The model under review builds one solid part; all positions refer to its coordinate system, in mm. Coordinates: 2 decimals unless noted, no trailing zeros. Write each loop counter-clockwise with the first axis right and the second up, starting at its lowest first coordinate (ties: lowest second). Pieces come first, ordered by that corner, then holes. Notation, with made-up numbers: M 39,-13 L 63,-13 A9 cw 63,-7 Z; hole C 83,25.5 d1. An arc over 180 degrees is marked long. Answer as CSV lines item,"result". Start each with the question number.
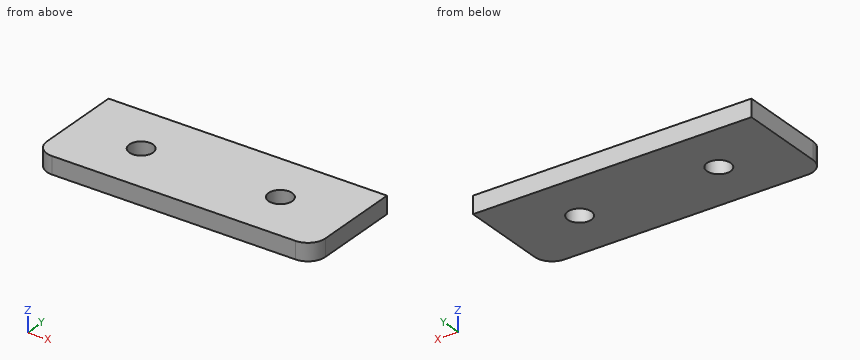
from build123d import *

# Parameters (mm, degrees)
IZIM1_W                     = 80
IZIM1_H                     = 30
Y_KSEKLIK_EKSTR_ZYON1_DEPTH = 5
RADYUS2_R                   = 5
IZIM2_R                     = 3.4
KES_EKSTR_ZYON1_DEPTH       = 8


with BuildPart() as part:
    # Çizim1 → Yükseklik-Ekstrüzyon1 (new body)
    with BuildSketch(Plane.XY):
        Rectangle(IZIM1_W, IZIM1_H)
    extrude(amount=Y_KSEKLIK_EKSTR_ZYON1_DEPTH)

    # Radyus2
    radyus2_edges = [part.edges().sort_by_distance(p)[0] for p in [
        (40, -15, 2.5),
        (-40, -15, 2.5),
    ]]
    fillet(radyus2_edges, radius=RADYUS2_R)

    # Çizim2 → Kes-Ekstrüzyon1 (cut)
    with BuildSketch(Plane.XY.offset(5)):
        with Locations((-20, 0)):
            Circle(IZIM2_R)
        with Locations((20, 0)):
            Circle(IZIM2_R)
    extrude(amount=-KES_EKSTR_ZYON1_DEPTH, mode=Mode.SUBTRACT)


solid = part.part
1) Take a section at A-A on x = 20. Give the boundary of the cut face in (y, z).
2) To check wall thickness, follow line 1 (Y direction, x = -20, z = 2.5); line 2 (X direction, y = 3, z = 0.5); line 3 (X direction, y = -2.5, z = 4.05). State the ranges of each line that lie inside material, in increasing order. Write a range as [from, to].
3) Clearance check with a flat-ended pin moving along its axis: pin 1 Ø2 at (x, y) = (0.5, 4) entering from -Z. State where the tip first meets the part, or that it passes through.
4) Take a section at C-C on y = 0. Give the boundary of the cut face in (x, z).
5) Take a section at B-B on z = 1.15. Give the boundary of the cut face in (x, y), and give its area (3 significant figures).
6) Take a section at D-D on x = -22. Give the boundary of the cut face in (y, z), and give its area (3 significant figures).
Results:
1,outline,"M -15,0 L -3.4,0 L -3.4,5 L -15,5 Z; M 3.4,0 L 15,0 L 15,5 L 3.4,5 Z"
2,line 1,"y = [-15, -3.4], [3.4, 15]"
2,line 2,"x = [-40, -21.6], [-18.4, 18.4], [21.6, 40]"
2,line 3,"x = [-40, -22.3], [-17.7, 17.7], [22.3, 40]"
3,pin 1,"stops at z = 0"
4,outline,"M -40,0 L -23.4,0 L -23.4,5 L -40,5 Z; M -16.6,0 L 16.6,0 L 16.6,5 L -16.6,5 Z; M 23.4,0 L 40,0 L 40,5 L 23.4,5 Z"
5,outline,"M -40,-10 A5 ccw -35,-15 L 35,-15 A5 ccw 40,-10 L 40,15 L -40,15 Z; hole C -20,0 d6.8; hole C 20,0 d6.8"
5,area,"2,320 mm²"
6,outline,"M -15,0 L -2.75,0 L -2.75,5 L -15,5 Z; M 2.75,0 L 15,0 L 15,5 L 2.75,5 Z"
6,area,"123 mm²"
